CAD build for the part. Positions are in the model's coordinates, mm. Round coordinates to 2 decimals unless told otherwise and drop trailing zeros. Loops run counter-clockwise (first coordinate to the right, second up) from the corner with the lowest first, then second, coordinate; pieces in that order, holes last.
Autodesk Inventor part; units mm, degrees
ref_plane "YZ Plane" through (0, 0, 0) normal (1, 0, 0) x (0, 1, 0)
ref_plane "XZ Plane" through (0, 0, 0) normal (0, 1, 0) x (-1, 0, 0)
ref_plane "XY Plane" through (0, 0, 0) normal (0, 0, 1) x (1, 0, 0)
sketch "Sketch1" plane through (0, 0, 0) normal (0, 1, 0) x (-1, 0, 0)
  point P0 (0, 0)
sketch "Sketch2" plane through (0, 0, 0) normal (0, 0, 1) x (1, 0, 0)
  line L0 (0, 0) -> (100, 0)
  line L1 (100, 0) -> (100, 30)
  line L2 (100, 30) -> (120, 60)
  line L3 (120, 60) -> (150, 60)
  line L4 (150, 60) -> (150, 80)
  line L5 (150, 80) -> (-50, 80)
  line L6 (-50, 80) -> (-50, 60)
  line L7 (0, 30) -> (0, 0)
  line L8 (-50, 60) -> (-20, 60)
  line L9 (-20, 60) -> (0, 30)
  dimension "d0" = 100
  dimension "d1" = 200
  dimension "d2" = 0
  dimension "d3" = 20
  dimension "d4" = 30
  dimension "d5" = 30
  dimension "d6" = 20
  dimension "d7" = 30
  dimension "d8" = 30
  dimension "d9" = 20
  dimension "d10" = 20
sketch "Sketch3" plane through (0, 0, 0) normal (0, 0, 1) x (1, 0, 0)
  point P0 (0, 0)
sketch "Sketch4" plane through (0, 0, 0) normal (0, 0, 1) x (1, 0, 0)
  point P0 (0, 0)
extrude "Extrusion1" add sketch "Sketch2" along normal blind 3
sketch "Sketch6" plane through (0, 0, 3) normal (0, 0, 1) x (1, 0, 0)
  point P0 (0, 0)
sketch "Sketch7" plane through (0, 0, 0) normal (0, 0, -1) x (-1, 0, 0)
  point P0 (0, 0)
sketch "Sketch8" plane through (0, 0, 3) normal (0, 0, 1) x (1, 0, 0)
  point P0 (0, 0)
sketch "Sketch9" plane through (0, 0, 3) normal (0, 0, 1) x (1, 0, 0)
  line L0 (-50, 80) -> (-50, 60)
  line L1 (150, 80) -> (-50, 80)
  line L2 (0, 30) -> (0, 0)
  line L3 (0, 0) -> (100, 0)
  point P0 (15, 16)
  point P1 (15, 7)
  dimension "d37" = 15
  dimension "d38" = 15
  dimension "d39" = 7
  dimension "d40" = 9
hole "Hole2" at (15, 7, 3) at (15, 16, 3) direction (0, 0, -1) diameter 3.4 end through all
sketch "Sketch11" plane through (0, 0, 3) normal (0, 0, 1) x (1, 0, 0)
  line L0 (100, 0) -> (100, 30)
  point P0 (0, 0)
sketch "Sketch12" plane through (0, 0, 3) normal (0, 0, 1) x (1, 0, 0)
  line L0 (-50, 80) -> (-50, 60)
  line L1 (150, 80) -> (-50, 80)
  point P0 (0, 0)
  point P1 (-41, 73)
  point P2 (-7, 73)
  dimension "d50" = 9
  dimension "d51" = 34
  dimension "d52" = 7
  dimension "d53" = 7
hole "Hole3" at (-41, 73, 3) at (-7, 73, 3) direction (0, 0, -1) diameter 4.4 end through all
ref_plane "Work Plane2" through (50, 0, 0) normal (-1, 0, 0) x (0, 0, 1)
mirror "Mirror1" about plane through (50, 0, 0) normal (-1, 0, 0) of "Hole2", "Hole3"
sketch "Sketch14" plane through (0, 0, 3) normal (0, 0, 1) x (1, 0, 0)
  point P0 (0, 0)
sketch "Sketch15" plane through (0, 0, 3) normal (0, 0, 1) x (1, 0, 0)
  point P0 (0, 0)
sketch "Sketch16" plane through (0, 0, 3) normal (0, 0, 1) x (1, 0, 0)
  point P0 (0, 0)
properties part number "plate"
Item 1: Probe line 1 (X direction, y = 7, z = 1); line 2 (Y direction, x = 15, z = 0.6); line 3 (X direction, y = 73, z = 1.9). List the from-to ranges inside material, lowest first.
Answers follow:
line 1: x = 0 to 13.3, 16.7 to 83.3, 86.7 to 100
line 2: y = 0 to 5.3, 8.7 to 14.3, 17.7 to 80
line 3: x = -50 to -43.2, -38.8 to -9.2, -4.8 to 104.8, 109.2 to 138.8, 143.2 to 150
Item 2: Flat gauge pins, fed straight in: P1, Ø0.9, axis at x = -29, z = 1.5, coming from the -Y side; P2, Ø0.9, axis at y = 18, z = 1.5, coming from the -X side; P3, Ø5.5, axis at x = 15, y = 16, coming from the +Z side. Where does each tip first touch, or does it go through?
Answers follow:
P1: stops at y = 60
P2: stops at x = 0
P3: stops at z = 3
Item 3: Cut at D-D, the plane x = 107. Give the cut face in (y, z).
Answers follow:
outline: (40.5, 0) - (70.8, 0) - (70.8, 3) - (40.5, 3) - close; (75.2, 0) - (80, 0) - (80, 3) - (75.2, 3) - close
Item 4: Two-plate mould, pull along X, no slides. Class faces 1 (the cylindrical face through (-39.05, 71.98, 1.48)), 2 (the flat face through (49, 49, 0)), 3 (the flat face through (-10, 45, 1)): released by +X, released by -X, zero draft, split by the parting line, or undercut.
Answers follow:
face 1: undercut
face 2: zero draft
face 3: released by -X
Item 5: Cut at B-B, the plane y = 73. Give the cut face in (x, z).
Answers follow:
outline: (-50, 0) - (-43.2, 0) - (-43.2, 3) - (-50, 3) - close; (-38.8, 0) - (-9.2, 0) - (-9.2, 3) - (-38.8, 3) - close; (-4.8, 0) - (104.8, 0) - (104.8, 3) - (-4.8, 3) - close; (109.2, 0) - (138.8, 0) - (138.8, 3) - (109.2, 3) - close; (143.2, 0) - (150, 0) - (150, 3) - (143.2, 3) - close
Item 6: Cut at C-C, the plane z = 0.6. State how many separate pieces and enclosed holes the cut face has, plus the area to 3 significant figures.
Answers follow:
separate pieces: 1
enclosed holes: 8
area: 10,500 mm2
Item 7: Cut at A-A, the plane x = -41. Give the cut face in (y, z).
Answers follow:
outline: (60, 0) - (70.8, 0) - (70.8, 3) - (60, 3) - close; (75.2, 0) - (80, 0) - (80, 3) - (75.2, 3) - close
